Check sheet for the modelled part. Datum: model origin and axes. Units: mm. Face numbers are marked on the shaded views. A direction names the side the tool comes from. Give positions to 0.01 mm unless a question says otherwise; leave off trailing zeros. Order: outer loops, then holes, each group sorted by start corner. A loop starts at its lowest first (then second) coordinate and runs counter-clockwise, first axis right, second up.
```python
from build123d import *

# Parameters (mm, degrees)
SKETCH_R        = 5
SKETCH_R_2      = 1.5
PAD_DEPTH       = 8
SKETCH029_W     = 10
SKETCH029_H     = 16
POCKET_DEPTH    = 8.001
SKETCH030_R     = 2.9
POCKET016_DEPTH = 3
CHAMFER_SIZE    = 1


with BuildPart() as part:
    # Sketch → Pad (new body)
    with BuildSketch(Plane.XY):
        with BuildLine():
            Line((-10.5, 16), (10.5, 16))
            ThreePointArc((16, 10.5), (14.389087, 14.389087), (10.5, 16))
            Line((16, 10.5), (16, -10.5))
            ThreePointArc((10.5, -16), (14.389087, -14.389087), (16, -10.5))
            Line((10.5, -16), (-10.5, -16))
            ThreePointArc((-16, -10.5), (-14.389087, -14.389087), (-10.5, -16))
            Line((-16, -10.5), (-16, 10.5))
            ThreePointArc((-10.5, 16), (-14.389087, 14.389087), (-16, 10.5))
        make_face()
        Circle(SKETCH_R, mode=Mode.SUBTRACT)
        with Locations((-10.5, 0)):
            Circle(SKETCH_R_2, mode=Mode.SUBTRACT)
        with Locations((10.5, 0)):
            Circle(SKETCH_R_2, mode=Mode.SUBTRACT)
    extrude(amount=PAD_DEPTH)

    # Sketch029 (on Face13 of Pad) → Pocket (cut, through all)
    with BuildSketch(Plane.XY.offset(8)):
        with Locations((0, -8)):
            Rectangle(SKETCH029_W, SKETCH029_H)
    extrude(amount=-POCKET_DEPTH, mode=Mode.SUBTRACT)

    # Sketch030 (on Face5 of Pocket) → Pocket016 (cut)
    with BuildSketch(Plane.XY.offset(8)):
        with Locations((-10.5, 0)):
            Circle(SKETCH030_R)
        with Locations((10.5, 0)):
            Circle(SKETCH030_R)
    extrude(amount=-POCKET016_DEPTH, mode=Mode.SUBTRACT)

    # Chamfer
    chamfer_edges = [part.edges().sort_by_distance(p)[0] for p in [
        (-14.389087, -14.389087, 8),
        (-16, 0, 8),
        (-7.75, -16, 8),
        (-14.389087, 14.389087, 8),
        (-5, -8, 8),
        (0, 16, 8),
        (0, 5, 8),
        (14.389087, 14.389087, 8),
        (5, -8, 8),
        (16, 0, 8),
        (7.75, -16, 8),
        (14.389087, -14.389087, 8),
        (7.6, 0, 8),
        (-13.4, 0, 8),
    ]]
    chamfer(chamfer_edges, length=CHAMFER_SIZE)


with BuildPart() as part_1:
    # Body placement: moved
    add(part.part.moved(Location((0, 0, 22))))


solid = part_1.part
```
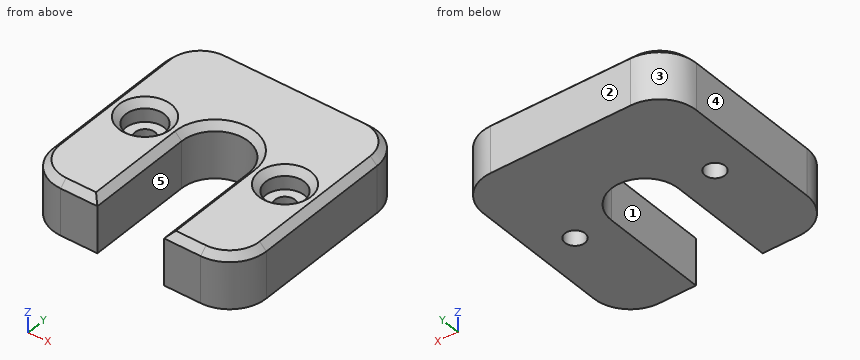
Q1. Tool access check on the marked faces 4 and 5. Record the directions out of +Z, -Z, +X, -X, +Y, -Y that give a thin tool (end or side, any length) a straight path to the whole face; none if there is none.
Q2. Sectioned sample at C-C, the plane z = 27.5. Record the cut outline in (x, y).
Q3. Material ranges on line 1 (X direction, y = 0, z = 25.6); line 2 (Y direction, x = 10.5, z = 24.1); line 3 (Y direction, x = -10.5, z = 28.2), recorded low to high.
Q4. Sectioned sample at D-D, the plane x = 0. Record the cut outline in (y, z).
Q5. Sectioned sample at A-A, the plane y = -10. Record the cut outline in (x, z).
Q6. Go/stop test with flat-tipped pins: P1, Ø3, axis at x = 11, y = -1, coming from the +Z side; P2, Ø6, axis at x = 8.5, y = 2, coming from the +Z side; P3, Ø6, axis at x = 2, y = 0.5, coming from the +Z side. Record where each tip stops, or that it passes through.
Q7. Draft check along X on the marked faces 1, 2 and 3. Enter one of: pulls with the +X half, pulls with the -X half, needs draft (parallel to the pull), parting line crosses it, or undercut.
Q8. Sectioned sample at B-B, the plane z = 23.5. Record the cut outline in (x, y).
Filled in:
1. face 4: +Z, -Z, -X, +Y, -Y
1. face 5: +Z, -Z, -Y
2. outline: (-16, -10.5) arc R5.5 ccw to (-10.5, -16) - (-5, -16) - (-5, 0) arc R5 cw to (5, 0) - (5, -16) - (10.5, -16) arc R5.5 ccw to (16, -10.5) - (16, 10.5) arc R5.5 ccw to (10.5, 16) - (-10.5, 16) arc R5.5 ccw to (-16, 10.5) - close; hole circle Ø5.8 at (-10.5, 0); hole circle Ø5.8 at (10.5, 0)
3. line 1: x = -16 to -12, -9 to -5, 5 to 9, 12 to 16
3. line 2: y = -16 to -1.5, 1.5 to 16
3. line 3: y = -16 to -2.9, 2.9 to 16
4. outline: (5, 22) - (16, 22) - (16, 29) - (15, 30) - (6, 30) - (5, 29) - close
5. outline: (-16, 22) - (-5, 22) - (-5, 29) - (-6, 30) - (-15, 30) - (-16, 29) - close; (5, 22) - (16, 22) - (16, 29) - (15, 30) - (6, 30) - (5, 29) - close
6. P1: stops at z = 27
6. P2: stops at z = 30
6. P3: stops at z = 29.06
7. face 1: undercut
7. face 2: needs draft
7. face 3: pulls with the -X half
8. outline: (-16, -10.5) arc R5.5 ccw to (-10.5, -16) - (-5, -16) - (-5, 0) arc R5 cw to (5, 0) - (5, -16) - (10.5, -16) arc R5.5 ccw to (16, -10.5) - (16, 10.5) arc R5.5 ccw to (10.5, 16) - (-10.5, 16) arc R5.5 ccw to (-16, 10.5) - close; hole circle Ø3 at (-10.5, 0); hole circle Ø3 at (10.5, 0)
